Design review of the part built by this model. Coordinates are the model's own, in mm. Face numbers are marked on the shaded views. A direction names the side the tool comes from. Round coordinates to 2 decimals unless told otherwise and drop trailing zeros. Loops run counter-clockwise (first coordinate to the right, second up) from the corner with the lowest first, then second, coordinate; pieces in that order, holes last. Notation, with made-up numbers: (-9.75, 32) - (45.25, 32) arc R35 cw to (45.25, 65) - close; hole circle Ø8 at (71, 63). An arc over 180 degrees is marked (long way). Return JSON: item names as keys, results as strings. Group by question number.
from build123d import *

# Parameters (mm, degrees)
SKETCH1_R           = 1.75
BOSS_EXTRUDE1_DEPTH = 10
BOSS_EXTRUDE2_DEPTH = 12
BOSS_EXTRUDE3_DEPTH = 22
CHAMFER1_SIZE       = 6


with BuildPart() as part:
    # Sketch1 → Boss-Extrude1 (new body)
    with BuildSketch(Plane(origin=(0, 0, 0), x_dir=(1, 0, 0), z_dir=(0, 1, 0))):
        with BuildLine():
            Line((-5, 22), (-5, 0))
            ThreePointArc((-5, 0), (0, -5), (5, 0))
            Line((5, 0), (5, 9))
            ThreePointArc((5, 9), (4, 10), (5, 11))
            Line((5, 11), (5, 22))
            Line((5, 22), (-5, 22))
        make_face()
        with Locations(Location((0, 0, 0), (0, 0, 270))):
            Circle(SKETCH1_R, mode=Mode.SUBTRACT)
    extrude(amount=BOSS_EXTRUDE1_DEPTH)

    # Sketch3 → Boss-Extrude2 (add)
    with BuildSketch(Plane(origin=(0, 10, 0), x_dir=(1, 0, 0), z_dir=(0, 1, 0))):
        with BuildLine():
            Line((5, 5.5), (-5, 5.5))
            Line((-5, 5.5), (-5, 22))
            Line((-5, 22), (5, 22))
            Line((5, 22), (5, 11))
            ThreePointArc((5, 11), (4, 10), (5, 9))
            Line((5, 9), (5, 5.5))
        make_face()
    extrude(amount=BOSS_EXTRUDE2_DEPTH)

    # Sketch5 → Boss-Extrude3 (add)
    with BuildSketch(Plane(origin=(0, 22, 0), x_dir=(1, 0, 0), z_dir=(0, 1, 0))):
        Polygon((5, 22), (5, 28), (1, 28), (-1, 25), (1, 25), (1, 22), align=None)
    extrude(amount=-BOSS_EXTRUDE3_DEPTH)

    # Chamfer1
    chamfer1_edges = [part.edges().sort_by_distance(p)[0] for p in [
        (-5, 11, -22),
    ]]
    chamfer(chamfer1_edges, length=CHAMFER1_SIZE - 0.0001)  # a hair under: the kernel refuses the full size


solid = part.part
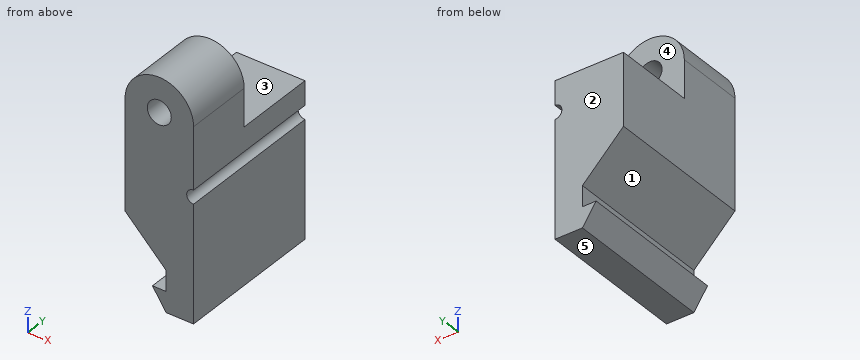
Q1. Draft analysis for pull direction Z (two halves, no side actions). For the marked faces 1, 2 and 3, state which applies: pulls with the +Z half, pulls with the -Z half, needs draft (parallel to the pull), parting line crosses it, or undercut.
Q2. For line 1 (Z direction, x = 2.75, y = 20.75); line 2 (X direction, y = 18.5, z = -21); line 3 (Y direction, x = -4, z = -1.5), list the stretches that pass through material, from the lowest coordinate up.
Q3. Add section D-D, the plane z = -2.5. State the section outline as (x, y) points.
Q4. Insertion check: pin 1 Ø5 at (x, y) = (2, 13) entering from +Z; pin 2 Ø3 at (x, z) = (0, 0) entering from -Y; pin 3 Ø6 at (x, z) = (0.5, -23.5) entering from +Y; pin 4 Ø2 at (x, y) = (-2.5, 15.5) entering from -Z. Each pin has a flat end and moves straight along its axis. Give the tip position at first contact, or say it passes through.
Q5. Add section B-B, the plane x = 0. State the section outline as (y, z) points, plus the area to 3 significant figures.
Q6. Tool access review of the marked faces 4 and 5: name each direction out of +Z, -Z, +X, -X, +Y, -Y from which nothing blocks a thin tool from reaching the whole face with its end or side.
Evaluation:
{
 "1": {"face 1": "undercut", "face 2": "needs draft", "face 3": "pulls with the +Z half"},
 "2": {"line 1": "-28 to -5.5", "line 2": "0 to 5", "line 3": "0 to 10"},
 "3": {"outline": "(-5, 0) - (5, 0) - (5, 10) - (-5, 10) - close"},
 "4": {"pin 1": "z = -5.5", "pin 2": "through", "pin 3": "y = 22", "pin 4": "z = -19.5"},
 "5": {"outline": "(0, -26.5) - (22, -26.5) - (22, -25) - (0, -25) - close; (0, -21) - (22, -21) - (22, -5.5) - (10, -5.5) - (10, -1.75) - (0, -1.75) - close; (0, 1.75) - (10, 1.75) - (10, 5) - (0, 5) - close", "area": "444 mm²"},
 "6": {"face 4": "+Z, +X, -X, +Y", "face 5": "-Z, +X, -X, +Y, -Y"}
}
